Autodesk Inventor part; units mm, degrees
ref_plane "YZ Plane" through (0, 0, 0) normal (1, 0, 0) x (0, 1, 0)
ref_plane "XZ Plane" through (0, 0, 0) normal (0, 1, 0) x (-1, 0, 0)
ref_plane "XY Plane" through (0, 0, 0) normal (0, 0, 1) x (1, 0, 0)
sketch "Sketch1" plane through (0, 0, 0) normal (0, 0, 1) x (1, 0, 0)
  line L0 (-16.8678, 0) -> (148.1322, 0)
  line L1 (-16.8678, 0) -> (-16.8678, 50)
  line L2 (-16.8678, 50) -> (148.1322, 50)
  line L3 (148.1322, 50) -> (148.1322, 0)
  line L4 (-16.8678, 0) -> (-16.8678, -3)
  line L5 (-16.8678, -3) -> (151.1322, -3)
  line L6 (151.1322, -3) -> (151.1322, 50)
  line L7 (151.1322, 50) -> (151.1322, 53)
  line L8 (151.1322, 53) -> (-19.8606, 54.5715)
  line L9 (-19.8606, 54.5715) -> (-20.3897, -3)
  arc A0 (-20.3897, -3) -> (-16.8678, -3) centre (-18.6288, 188.6018) ccw
  point P0 (0, 0)
  dimension "d0" = 165
  dimension "d2" = 50
  dimension "d3" = 165
  dimension "d4" = 3
  dimension "d5" = 168
  dimension "d6" = 53
  dimension "d7" = 3
  dimension "d8" = 171
extrude "Extrusion1" add sketch "Sketch1" along normal blind 100
sketch "Sketch2" plane through (0, 0, 100) normal (0, 0, 1) x (1, 0, 0)
  line L0 (148.1322, 0) -> (-16.8678, 0)
  line L1 (-16.8678, 0) -> (-1.8678, 0)
  line L2 (-1.8678, 0) -> (-1.8678, 3.4426)
  line L3 (-1.8678, 0) -> (-1.8678, 25)
  line L4 (-1.8678, 25) -> (133.1322, 25)
  line L5 (133.1322, 25) -> (133.1322, 0)
  line L6 (-16.8678, 0) -> (-16.8678, 50)
  line L7 (-16.8678, 50) -> (148.1322, 50)
  line L8 (148.1322, 50) -> (148.1322, 0)
  line L9 (148.1322, 0) -> (133.1322, 0)
  point P0 (0, 0)
  dimension "d11" = 15
  dimension "d12" = 25
  dimension "d13" = 135
  dimension "d14" = 50
  dimension "d15" = 165
  dimension "d16" = 50
extrude "Extrusion2" add sketch "Sketch2" against normal blind 3 contours L0 L5 L4 L3 L2 L6 L7 L8
sketch "Sketch3" plane through (0, 0, 0) normal (0, 0, -1) x (-1, 0, 0)
  line L0 (-148.1322, 0) -> (16.8678, 0)
  line L1 (-148.1322, 0) -> (16.8678, 0)
  line L2 (16.8678, 0) -> (16.8678, 50)
  line L3 (16.8678, 50) -> (-148.1322, 50)
  line L4 (-148.1322, 50) -> (-148.1322, 0)
  point P0 (0, 0)
  dimension "d19" = 165
  dimension "d20" = 50
  dimension "d21" = 165
extrude "Extrusion3" add sketch "Sketch3" against normal blind 3
sketch "Sketch4" plane through (151.1322, -3, 0) normal (1, 0, 0) x (0, 0, -1)
  line L0 (-32.782, 20.9659) -> (-8.782, 20.9659)
  line L1 (-8.782, 20.9659) -> (-8.782, 5.9659)
  line L2 (-8.782, 5.9659) -> (-32.782, 5.9659)
  line L3 (-32.782, 5.9659) -> (-32.782, 20.9659)
  point P0 (0, 3)
  dimension "d24" = 24
  dimension "d25" = 15
extrude "Extrusion4" cut sketch "Sketch4" against normal blind 3
properties part number "Main"
Source: CAD feature listing. Evaluate the final solid. Frame: model axes, mm. A direction names the side the tool comes from. Give positions to 0.01 mm unless a question says otherwise; leave off trailing zeros. Write each loop counter-clockwise with the first axis right and the second up, starting at its lowest first coordinate (ties: lowest second). Pieces come first, ordered by that corner, then holes. Notation, with made-up numbers: M -16,-28.75 L 33,-28.75 A12 ccw 33,-21.75 Z; hole C 72,59.5 d10. An arc over 180 degrees is marked long. Return JSON: item names as keys, results as strings. Group by question number.
1) Cut plane B-B, the plane y = 34.5. Output: boundary loops of the cut face in (x, z).
2) Cut plane D-D, the plane x = 87. Output: boundary loops of the cut face in (y, z).
3) Cut plane A-A, the plane z = 6.5. Output: boundary loops of the cut face in (x, y).
4) Cut plane C-C, the plane y = 10. Output: boundary loops of the cut face in (x, z).
5) Draft query along Z for faces 1 (the face through (148.132, 25, 49)), 2 (the face through (64, 33, 100)), 3 (the face through (151.132, 25, 49)). Return one class per face: released by +Z, released by -Z, zero draft, split by the parting line, or undercut.
6) Set-up query: faces 4 (the face through (66, -3, 49)), 5 (the face through (64, 0, 51)). Return all of +Z, -Z, +X, -X, +Y, -Y with unobstructed straight access to the full face (end or side cutting, diameter ignored); none if empty.
7) First-contact query: pin 1 Ø2 at (x, z) = (65, 66.5) entering from +Y; pin 2 Ø6 at (x, z) = (62.5, 86) entering from -Y; pin 3 Ø0.9 at (y, z) = (11, 98) entering from -X. Flat tips, straight axial feed; report the tip coordinate or a pass-through.
8) Ray query, L1, parallel to Z at x = 87, y = 45.5; L2, parallel to X at y = 1, z = 16.5; L3, parallel to X at y = 5.5, z = 7. Return the intervals inside material, ascending.
Data:
{
 "1": {"outline": "M -20.05,0 L 151.13,0 L 151.13,100 L -20.05,100 Z; hole M -16.87,3 L 148.13,3 L 148.13,97 L -16.87,97 Z"},
 "2": {"outline": "M -3,0 L 53.59,0 L 53.59,100 L 25,100 L 25,97 L 50,97 L 50,3 L 0,3 L 0,100 L -3,100 Z"},
 "3": {"outline": "M -20.39,-3 A191.62 ccw -16.87,-3 L 151.13,-3 L 151.13,53 L -19.86,54.57 Z; hole M -16.87,0 L 148.13,0 L 148.13,50 L -16.87,50 Z"},
 "4": {"outline": "M -20.27,0 L 151.13,0 L 151.13,8.78 L 148.13,8.78 L 148.13,3 L -16.87,3 L -16.87,97 L -1.87,97 L -1.87,100 L -20.27,100 Z; M 133.13,97 L 148.13,97 L 148.13,32.78 L 151.13,32.78 L 151.13,100 L 133.13,100 Z"},
 "5": {"face 1": "undercut", "face 2": "released by +Z", "face 3": "zero draft"},
 "6": {"face 4": "+Z, -Z, +X, -X, -Y", "face 5": "none"},
 "7": {"pin 1": "stops at y = 53.8", "pin 2": "stops at y = -3", "pin 3": "stops at x = -20.27"},
 "8": {"L1": "z = 0 to 3, 97 to 100", "L2": "x = -20.35 to -16.87, 148.13 to 151.13", "L3": "x = -20.31 to -16.87, 148.13 to 151.13"}
}
